from build123d import *

# Parameters (mm, degrees)
SKETCH1_R           = 3.175
BOSS_EXTRUDE1_DEPTH = 203.2
SKETCH2_W           = 2.54
SKETCH2_H           = 2.54
BOSS_EXTRUDE2_DEPTH = 12.7


with BuildPart() as part:
    # Sketch1 → Boss-Extrude1 (new body)
    with BuildSketch(Plane.XY):
        Circle(SKETCH1_R)
    extrude(amount=BOSS_EXTRUDE1_DEPTH)

    # Sketch2 → Boss-Extrude2 (add)
    with BuildSketch(Plane(origin=(0, 0, 0), x_dir=(1, 0, 0), z_dir=(0, 1, 0))):
        with Locations((0.323252362, -106.68)):
            Rectangle(SKETCH2_W, SKETCH2_H)
        with Locations((0.323252362, -125.73)):
            Rectangle(SKETCH2_W, SKETCH2_H)
        with Locations((0.323252362, -87.63)):
            Rectangle(SKETCH2_W, SKETCH2_H)
        with Locations((0.323252362, -68.58)):
            Rectangle(SKETCH2_W, SKETCH2_H)
    extrude(amount=BOSS_EXTRUDE2_DEPTH)


solid = part.part
Part model, mm, in its own coordinate system. Give positions to 0.01 mm unless a question says otherwise; leave off trailing zeros. Order: outer loops, then holes, each group sorted by start corner. A loop starts at its lowest first (then second) coordinate and runs counter-clockwise, first axis right, second up. Notation, with made-up numbers: (61.25, 39) - (109.25, 39) arc R13 ccw to (109.25, 48) - close; hole circle Ø7 at (-38.5, 52). An arc over 180 degrees is marked (long way). Use a Markdown table: item, result.
1) Saw through at A-A on y = 5.75. List the corners of the cut face in (x, z), plus the area to 3 significant figures.
Checked values:
| item | result |
|---|---|
| outline | (-0.95, 67.31) - (1.59, 67.31) - (1.59, 69.85) - (-0.95, 69.85) - close; (-0.95, 86.36) - (1.59, 86.36) - (1.59, 88.9) - (-0.95, 88.9) - close; (-0.95, 105.41) - (1.59, 105.41) - (1.59, 107.95) - (-0.95, 107.95) - close; (-0.95, 124.46) - (1.59, 124.46) - (1.59, 127) - (-0.95, 127) - close |
| area | 25.8 mm² |
2) Flat gauge pins, fed straight in: P1, Ø2, axis at x = 0, y = 7, coming from the +Z side; P2, Ø2, axis at y = 7, z = 68.5, coming from the +X side; P3, Ø0.8, axis at x = 0, y = 5.5, coming from the -Z side. Where does each tip first touch, or does it go through?
Checked values:
| item | result |
|---|---|
| P1 | z = 127 |
| P2 | x = 1.59 |
| P3 | z = 67.31 |
3) Saw through at B-B on z = 122. List the corners of the cut face in (x, y) (3 decimals), plus the area to 3 significant figures.
Checked values:
| item | result |
|---|---|
| outline | circle Ø6.35 at (0, 0) |
| area | 31.7 mm² |
4) Probe L1, parallel to Z at x = 1.5, y = 4.25; L2, parallel to X at y = -0.25, z = 158; L3, parallel to Y at x = 0.5, z = 191. List the from-to ranges inside material, lowest first. Write a range as from..to.
Checked values:
| item | result |
|---|---|
| L1 | 67.31..69.85, 86.36..88.9, 105.41..107.95, 124.46..127 |
| L2 | -3.17..3.17 |
| L3 | -3.14..3.14 |
